Verification items for the finished model (mm, model axes). Face numbers are marked on the shaded views. A direction names the side the tool comes from. Round coordinates to 2 decimals unless told otherwise and drop trailing zeros. Order: outer loops, then holes, each group sorted by start corner. A loop starts at its lowest first (then second) coordinate and runs counter-clockwise, first axis right, second up. Notation, with made-up numbers: (18.5, 16) -> (70.5, 16) arc R18 cw to (70.5, 23) -> close; hole circle Ø10 at (4, 3). An arc over 180 degrees is marked (long way). Put each result on its own line as item: value.
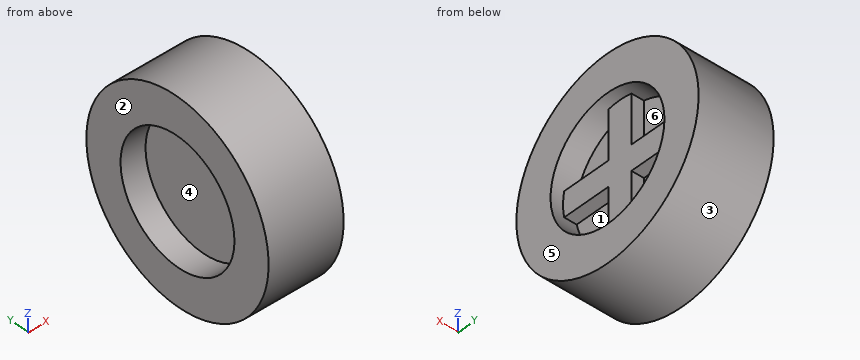
from build123d import *

# Parameters (mm, degrees)
SKETCH_1_R          = 4
EXTRUDE_1_DEPTH     = 3
SKETCH_2_R          = 2.5
CUT_EXTRUDE_1_DEPTH = 1
CUT_EXTRUDE_START   = -1
SKETCH_3_R          = 2.5
CUT_EXTRUDE_2_DEPTH = 1
EXTRUDE_START       = 0.5
EXTRUDE_2_DEPTH     = 0.5


with BuildPart() as part:
    # 草图1 → 凸台-拉伸1 (new body)
    with BuildSketch(Plane(origin=(0, 0, 0), x_dir=(0, 0, -1), z_dir=(1, 0, 0))):
        Circle(SKETCH_1_R)
    extrude(amount=EXTRUDE_1_DEPTH)

    # 草图2 → 切除-拉伸1 (cut)
    with BuildSketch(Plane(origin=(3, 0, 0), x_dir=(0, 0, -1), z_dir=(1, 0, 0))):
        Circle(SKETCH_2_R)
    extrude(amount=-CUT_EXTRUDE_1_DEPTH, mode=Mode.SUBTRACT)

    # 草图3 → 切除-拉伸2 (cut)
    with BuildSketch(Plane.ZY.offset(CUT_EXTRUDE_START)):
        with Locations(Location((0, 0, 0), (0, 0, 180))):
            Circle(SKETCH_3_R)
    extrude(amount=CUT_EXTRUDE_2_DEPTH, mode=Mode.SUBTRACT)

    # 草图4 → 凸台-拉伸2 (add)
    with BuildSketch(Plane(origin=(2, 0, 0), x_dir=(0, 0, -1), z_dir=(1, 0, 0)).offset(EXTRUDE_START)):
        with BuildLine():
            Line((-0.5, -0.5), (-0.5, -2.449489743))
            ThreePointArc((-0.5, -2.449489743), (0, -2.5), (0.5, -2.449489743))
            Line((0.5, -2.449489743), (0.5, -0.5))
            Line((0.5, -0.5), (2.449489743, -0.5))
            ThreePointArc((2.449489743, -0.5), (2.5, 0), (2.449489743, 0.5))
            Line((2.449489743, 0.5), (0.5, 0.5))
            Line((0.5, 0.5), (0.5, 2.449489743))
            ThreePointArc((0.5, 2.449489743), (0, 2.5), (-0.5, 2.449489743))
            Line((-0.5, 2.449489743), (-0.5, 0.5))
            Line((-0.5, 0.5), (-2.449489743, 0.5))
            ThreePointArc((-2.449489743, 0.5), (-2.5, 0), (-2.449489743, -0.5))
            Line((-2.449489743, -0.5), (-0.5, -0.5))
        make_face()
    extrude(amount=-EXTRUDE_2_DEPTH)


solid = part.part
Item 1: Tool access check on the marked faces 4, 5 and 6. Record the directions out of +Z, -Z, +X, -X, +Y, -Y that give a thin tool (end or side, any length) a straight path to the whole face; none if there is none.
Check sheet entries:
face 4: -X
face 5: +Z, -Z, +X, +Y, -Y
face 6: +X
Item 2: Release check for a two-part mould opening along Y. For the marked faces 1, 2 and 3 record: +Y half, -Y half, draft (parallel to the pull), parting line (faces both ways), or undercut.
Check sheet entries:
face 1: undercut
face 2: draft
face 3: parting line
Item 3: Gauge pin test, flat ends, axial feed: pin 1 Ø1.5 at (x, y) = (1, -0.5) entering from -Z; pin 2 Ø0.6 at (x, z) = (2, 2) entering from +Y; pin 3 Ø1.6 at (y, z) = (-1, 1) entering from +X; pin 4 Ø4.5 at (y, z) = (0, 0) entering from -X. Record the tip position at first contact, or that the pin passes through.
Check sheet entries:
pin 1: stops at z = -4
pin 2: stops at y = 3.62
pin 3: stops at x = 2.5
pin 4: stops at x = 1
Item 4: Section check D-D on x = 2.75. Record the boundary of the cut face in (y, z), then the cut area to 3 significant figures.
Check sheet entries:
outline: circle Ø8 at (0, 0); hole circle Ø5 at (0, 0)
area: 30.6 mm^2
Item 5: Section check B-B on y = 0. Record the boundary of the cut face in (x, z), then the cut area to 3 significant figures.
Check sheet entries:
outline: (0, -4) -> (3, -4) -> (3, -2.5) -> (2.5, -2.5) -> (2.5, 2.5) -> (3, 2.5) -> (3, 4) -> (0, 4) -> (0, 2.5) -> (1, 2.5) -> (1, -2.5) -> (0, -2.5) -> close
area: 16.5 mm^2
Item 6: Section check A-A on x = 2.25. Record the boundary of the cut face in (y, z), then the cut area to 3 significant figures.
Check sheet entries:
outline: circle Ø8 at (0, 0); hole (-2.45, -0.5) arc R2.5 ccw to (-0.5, -2.45) -> (-0.5, -0.5) -> close; hole (-2.45, 0.5) -> (-0.5, 0.5) -> (-0.5, 2.45) arc R2.5 ccw to start; hole (0.5, -2.45) arc R2.5 ccw to (2.45, -0.5) -> (0.5, -0.5) -> close; hole (0.5, 0.5) -> (2.45, 0.5) arc R2.5 ccw to (0.5, 2.45) -> close
area: 39.6 mm^2
Item 7: Material ranges on L1, parallel to Y at x = 2.65, z = 0; L2, parallel to Z at x = 0.65, y = -0.25; L3, parallel to Y at x = 0.5, z = -0.75, recorded low to high. Write a range as [from, to].
Check sheet entries:
L1: y = [-4, -2.5], [2.5, 4]
L2: z = [-3.99, -2.49], [2.49, 3.99]
L3: y = [-3.93, -2.38], [2.38, 3.93]
